from build123d import *

# Parameters (mm, degrees)
SKETCH1_R           = 6.35
BASE_EXTRUDE_DEPTH  = 38.1
SKETCH3_R           = 9.525
BOSS_EXTRUDE1_DEPTH = 15.875
CUT_EXTRUDE1_DEPTH  = 12.7
FILLET1_R           = 4.7625
FILLET2_R           = 4.7625
SKETCH5_R           = 1.190625
CUT_EXTRUDE2_DEPTH  = 42.790769119
CUT_EXTRUDE3_START  = -6.35
CUT_EXTRUDE3_DEPTH  = 6.35
CHAMFER1_SIZE       = 0.79375


with BuildPart() as part:
    # Sketch1 → Base-Extrude (new body)
    with BuildSketch(Plane(origin=(0, 0, 0), x_dir=(-1, 0, 0), z_dir=(0, 1, 0))):
        with Locations(Location((0, 0, 0), (0, 0, 270))):
            Circle(SKETCH1_R)
    extrude(amount=BASE_EXTRUDE_DEPTH)

    # Sketch3 → Boss-Extrude1 (add)
    with BuildSketch(Plane(origin=(0, 0, 0), x_dir=(-1, 0, 0), z_dir=(0, 1, 0))):
        with Locations(Location((0, 0, 0), (0, 0, 90))):
            Circle(SKETCH3_R)
    extrude(amount=BOSS_EXTRUDE1_DEPTH)

    # Sketch4 → Cut-Extrude1 (cut)
    with BuildSketch(Plane(origin=(0, 0, 0), x_dir=(-1, 0, 0), z_dir=(0, 1, 0))):
        with BuildLine():
            Line((-4.7625, 4.200130206), (-4.7625, -4.200130206))
            ThreePointArc((-4.7625, -4.200130206), (6.35, 0), (-4.7625, 4.200130206))
        make_face()
    extrude(amount=CUT_EXTRUDE1_DEPTH, mode=Mode.SUBTRACT)

    # Fillet1
    # the kernel refuses this fillet: 4.7625 mm, written as the material it adds along each edge
    with BuildSketch(Plane(origin=(0, 15.875, 0), x_dir=(0, 0, -1), z_dir=(-1, 0, 0))) as fillet1_piece_1:
        with BuildLine():
            CenterArc((11.1125, -4.490128061), FILLET1_R, 109.471220634, 70.528779366)
            Line((6.35, -4.490128061), (6.25475, -4.490128061))
            Line((6.25475, -4.490128061), (6.25475, 0))
            Line((6.25475, 0), (6.35, 0.09525))
            ThreePointArc((6.35, 0.09525), (7.9375, 0.09525), (9.49325, 0.089802561))
            Line((9.49325, 0.089802561), (9.525, 0))
        make_face()
    revolve(axis=Axis((0, 15.875, 0), (0, -1, 0)))

    # Fillet2
    fillet2_edges = [part.edges().sort_by_distance(p)[0] for p in [
        (9.525, 15.875, 0),
    ]]
    fillet(fillet2_edges, radius=FILLET2_R)

    # Sketch5 → Cut-Extrude2 (cut, through all)
    with BuildSketch(Plane.ZY.offset(-4.7625)):
        with Locations((0, 6.35)):
            Circle(SKETCH5_R)
    extrude(amount=-CUT_EXTRUDE2_DEPTH, mode=Mode.SUBTRACT)

    # Sketch7 → Cut-Extrude3 (cut)
    with BuildSketch(Plane(origin=(0, 38.1, 0), x_dir=(-1, 0, 0), z_dir=(0, 1, 0)).offset(CUT_EXTRUDE3_START)):
        with BuildLine():
            Line((-4.7625, 4.200130206), (-4.7625, -4.200130206))
            ThreePointArc((-4.7625, -4.200130206), (-6.35, 0), (-4.7625, 4.200130206))
        make_face()
    extrude(amount=CUT_EXTRUDE3_DEPTH, mode=Mode.SUBTRACT)

    # Chamfer1
    chamfer1_edges = [part.edges().sort_by_distance(p)[0] for p in [
        (-5.787630206, 38.1, 2.612630206),
    ]]
    chamfer(chamfer1_edges, length=CHAMFER1_SIZE)


solid = part.part
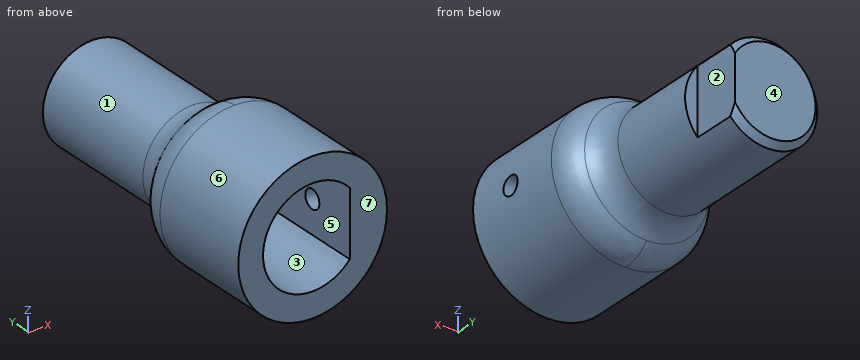
Design review of the part built by this model. Coordinates are the model's own, in mm. Face numbers are marked on the shaded views. A direction names the side the tool comes from. Give positions to 0.01 mm unless a question says otherwise; leave off trailing zeros. Loops run counter-clockwise (first coordinate to the right, second up) from the corner with the lowest first, then second, coordinate; pieces in that order, holes last. Notation, with made-up numbers: (57.25, 69.5) - (103.25, 69.5) arc R22 cw to (103.25, 80.5) - close; hole circle Ø2 at (-17, 86.25). An arc over 180 degrees is marked (long way). Write item = value, one per line.
1) Clearance check with flat-ended pins moving along their axes: pin 1 Ø9 at (x, z) = (1, 1.5) entering from -Y; pin 2 Ø5 at (y, z) = (34.5, 2) entering from +X; pin 3 Ø0.8 at (x, z) = (5.5, 2) entering from +Y; pin 4 Ø5 at (x, y) = (3.5, 14) entering from +Z. State where each tip first meets the part, or that it passes through.
Result sheet:
pin_1 = 0
pin_2 = 4.76
pin_3 = 31.75
pin_4 = 9.46
2) Draft analysis for pull direction Z (two halves, no side actions). For the marked faces 5, 6 and 7, state which applies: +Z half, -Z half, draft (parallel to the pull), parting line (faces both ways), or undercut.
Result sheet:
face_5 = undercut
face_6 = parting line
face_7 = draft
3) To check wall thickness, follow line 1 (X direction, y = 3.5, z = -2.25); line 2 (X direction, y = 2, z = 0.25); line 3 (Y direction, x = 7, z = 0.25). State the ranges of each line that lie inside material, in increasing order.
Result sheet:
line_1 = -9.26 to -5.94, 4.76 to 9.26
line_2 = -9.52 to -6.35, 4.76 to 9.52
line_3 = 0 to 5.19, 7.51 to 17.96
4) Take a section at B-B on y = 30. State the section outline as (x, z) points.
Result sheet:
outline = circle Ø12.7 at (0, 0)
5) Tool access review of the marked faces 1, 2, 3 and 4: name each direction out of +Z, -Z, +X, -X, +Y, -Y from which nothing blocks a thin tool from reaching the whole face with its end or side.
Result sheet:
face_1 = +Y
face_2 = +Z, -Z, +X, +Y
face_3 = -Y
face_4 = +Z, -Z, +X, -X, +Y
